from build123d import *

# Parameters (mm, degrees)
ESBO_O1_W                = 45
ESBO_O1_H                = 45
ESBO_O1_R                = 1.75
ESBO_O1_R_2              = 11.5
RESSALTO_EXTRUS_O1_DEPTH = 5
ESBO_O3_R                = 4
RESSALTO_EXTRUS_O2_DEPTH = 45


with BuildPart() as part:
    # Esboço1 → Ressalto-extrusão1 (new body)
    with BuildSketch(Plane.XY):
        Rectangle(ESBO_O1_W, ESBO_O1_H)
        with Locations((-15.5, 15.5)):
            Circle(ESBO_O1_R, mode=Mode.SUBTRACT)
        with Locations((15.5, 15.5)):
            Circle(ESBO_O1_R, mode=Mode.SUBTRACT)
        with Locations((15.5, -15.5)):
            Circle(ESBO_O1_R, mode=Mode.SUBTRACT)
        with Locations((-15.5, -15.5)):
            Circle(ESBO_O1_R, mode=Mode.SUBTRACT)
        Circle(ESBO_O1_R_2, mode=Mode.SUBTRACT)
    extrude(amount=RESSALTO_EXTRUS_O1_DEPTH)

    # Esboço3 → Ressalto-extrusão2 (add)
    # profile 1 of 2: a face of its own
    with BuildSketch(Plane.ZY.offset(22.5)):
        with BuildLine():
            Line((0, 30), (0, 21.937742252))
            Line((0, 21.937742252), (5, 21.937742252))
            ThreePointArc((5, 21.937742252), (16.64852927, 34.74341649), (0, 30))
        make_face()
        with Locations(Location((9, 30, 0), (0, 0, 270))):
            Circle(ESBO_O3_R, mode=Mode.SUBTRACT)
    # profile 2 of 2: a face of its own
    with BuildSketch(Plane.ZY.offset(22.5)):
        with BuildLine():
            Line((5, -21.937742252), (0, -21.937742252))
            Line((0, -21.937742252), (0, -30))
            ThreePointArc((0, -30), (16.64852927, -34.74341649), (5, -21.937742252))
        make_face()
        with Locations(Location((9, -30, 0), (0, 0, 270))):
            Circle(ESBO_O3_R, mode=Mode.SUBTRACT)
    extrude(amount=-RESSALTO_EXTRUS_O2_DEPTH)


solid = part.part
Can you work these out from the model? Positions are in its coordinate system, mm. Round coordinates to 2 decimals unless told otherwise and drop trailing zeros. Write each loop counter-clockwise with the first axis right and the second up, starting at its lowest first coordinate (ties: lowest second). Pieces come first, ordered by that corner, then holes. Notation, with made-up numbers: (59, -6.75) - (112, -6.75) arc R28 cw to (112, 13.25) - close; hole circle Ø11 at (6.5, 1.5). An arc over 180 degrees is marked (long way). Write each question's results on one line, items separated by ' | '. Start each with the question number.
1) Please list where these lines run through material, in increasing order: line 1 (Y direction, x = -11, z = 8.5); line 2 (Y direction, x = -15.5, z = 2.1); line 3 (Z direction, x = -6, y = -15.5).
2) Suppose I cut it at B-B (x = -15.5). List the corners of the cut face in (y, z) for me.
3) Suppose I cut it at A-A (x = 0). List the corners of the cut face in (y, z) for me.
4) For pin 1 Ø1 at (x, y) = (-16, -7) entering from +Z; pin 2 Ø1 at (x, y) = (-2.5, -17) entering from -Z; pin 3 Ø5 at (x, z) = (-4.5, 3.5) entering from +Y, each with a flat end and sliding along its axis, tell me the tip position at first contact or that it passes through.
5) We'd pull the mould along X, two halves only. Please class faces 1 (the cylindrical face through (-0.32, -35.02, 16.47)), 2 (the cylindrical face through (-14.6, -14, 2.5)), 3 (the flat face through (-22.5, 1, 3)): released by +X, released by -X, zero draft, split by the parting line, or undercut.
6) Suppose I cut it at D-D (y = 0). List the corners of the cut face in (x, z) for me, and give its area (3 significant figures).
7) Suppose I cut it at C-C (z = 9). List the corners of the cut face in (x, y) for me.
Here are the results:
1) line 1: y = -38.99 to -33.97, -26.03 to -21.01, 21.01 to 26.03, 33.97 to 38.99 | line 2: y = -35.78 to -17.25, -13.75 to 13.75, 17.25 to 35.78 | line 3: z = 0 to 5
2) outline: (-30, 0) - (-17.25, 0) - (-17.25, 5) - (-21.94, 5) arc R9 ccw (long way) to start; (-13.75, 0) - (13.75, 0) - (13.75, 5) - (-13.75, 5) - close; (17.25, 0) - (30, 0) arc R9 ccw (long way) to (21.94, 5) - (17.25, 5) - close; hole circle Ø8 at (-30, 9); hole circle Ø8 at (30, 9)
3) outline: (-30, 0) - (-11.5, 0) - (-11.5, 5) - (-21.94, 5) arc R9 ccw (long way) to start; (11.5, 0) - (30, 0) arc R9 ccw (long way) to (21.94, 5) - (11.5, 5) - close; hole circle Ø8 at (-30, 9); hole circle Ø8 at (30, 9)
4) pin 1: stops at z = 5 | pin 2: stops at z = 0 | pin 3: stops at y = 38.49
5) face 1: zero draft | face 2: undercut | face 3: released by -X
6) outline: (-22.5, 0) - (-11.5, 0) - (-11.5, 5) - (-22.5, 5) - close; (11.5, 0) - (22.5, 0) - (22.5, 5) - (11.5, 5) - close | area: 110 mm2
7) outline: (-22.5, -39) - (22.5, -39) - (22.5, -34) - (-22.5, -34) - close; (-22.5, -26) - (22.5, -26) - (22.5, -21) - (-22.5, -21) - close; (-22.5, 21) - (22.5, 21) - (22.5, 26) - (-22.5, 26) - close; (-22.5, 34) - (22.5, 34) - (22.5, 39) - (-22.5, 39) - close
